For this review, take the finished solid that the model builds, in its own axes (mm). Face numbers are marked on the shaded views. A direction names the side the tool comes from. Round coordinates to 2 decimals unless told otherwise and drop trailing zeros. Loops run counter-clockwise (first coordinate to the right, second up) from the corner with the lowest first, then second, coordinate; pieces in that order, holes last.
1. Consider section B-B on x = 5. State the section outline as (y, z) points, then the cut area to 3 significant figures.
2. Consider section A-A on y = 4. State the section outline as (x, z) points.
3. Clearance check with flat-ended pins moving along their axes: pin 1 Ø1.9 at (x, z) = (11, 2.5) entering from +Y; pin 2 Ø1.9 at (y, z) = (-38.5, 2.5) entering from -X; pin 3 Ø2 at (x, y) = (83, -19.5) entering from +Z; pin 4 Ø1 at (x, z) = (44.5, 3) entering from +Y. State where each tip first meets the part, or that it passes through.
4. To check wall thickness, follow line 1 along Y through (x, z) = (103.75, 0.25); line 2 along Z through (x, y) = (98, 2); line 3 along Y through (x, z) = (84, 2.75). State the ranges of each line that lie inside material, in increasing order.
5. Tool access review of the marked faces 1 and 2: name each direction out of +Z, -Z, +X, -X, +Y, -Y from which nothing blocks a thin tool from reaching the whole face with its end or side.
6. Consider section C-C on y = -37. State how many separate pieces and enclosed holes the cut face has, then the cut area to 3 significant figures.
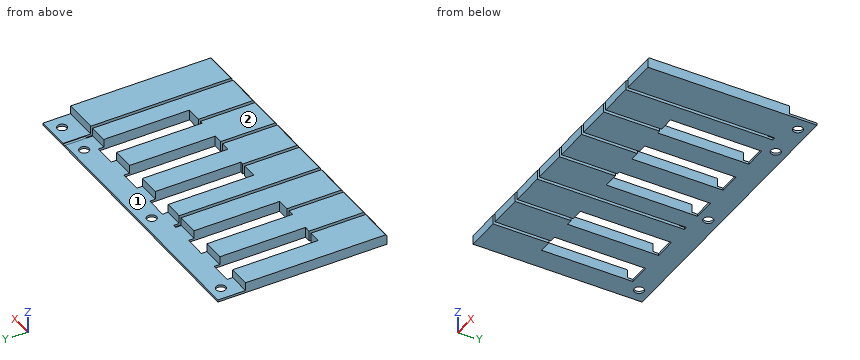
from build123d import *

# Parameters (mm, degrees)
PAD_DEPTH       = 0.81
SKETCH001_W     = 12.5
SKETCH001_H     = 51.2
PAD001_DEPTH    = 3
SKETCH002_R     = 1.75
POCKET_DEPTH    = 5
SKETCH003_W     = 1.25
SKETCH003_H     = 8
POCKET001_DEPTH = 0.2
CHAMFER_SIZE    = 0.5


with BuildPart() as part:
    # Sketch → Pad (new body)
    with BuildSketch(Plane.XY):
        Polygon((0, 0), (0, -53.2), (12.5, -53.2), (12.5, -33), (8, -33), (8, 0), (16, 0), (16, -33), (13.75, -33), (13.75, -53.2), (26.25, -53.2), (26.25, -33), (24, -33), (24, 0), (32, 0), (32, -33), (27.5, -33), (27.5, -53.2), (40, -53.2), (40, 0), (41.25, 0), (41.25, -53.2), (53.75, -53.2), (53.75, -33), (48.125, -33), (48.125, 0), (56.125, 0), (56.125, -33), (55, -33), (55, -53.2), (67.5, -53.2), (67.5, -33), (64.125, -33), (64.125, 0), (72.125, 0), (72.125, -33), (68.75, -33), (68.75, -53.2), (81.25, -53.2), (81.25, -33), (80.125, -33), (80.125, 0), (88.125, 0), (88.125, -33), (82.5, -33), (82.5, -53.2), (95, -53.2), (95, 0), (96.25, 0), (96.25, -53.2), (108.75, -53.2), (108.75, 0), (108.75, 8), (0, 8), align=None)
    extrude(amount=PAD_DEPTH)

    # Sketch001 (on Face56 of Pad) → Pad001 (join)
    with BuildSketch(Plane.XY.offset(0.81)):
        Polygon((0, -2), (0, -53.2), (12.5, -53.2), (12.5, -33), (8, -33), (8, -2), align=None)
        Polygon((16, -2), (16, -33), (13.75, -33), (13.75, -53.2), (26.25, -53.2), (26.25, -33), (24, -33), (24, -2), align=None)
        Polygon((32, -2), (32, -33), (27.5, -33), (27.5, -53.2), (40, -53.2), (40, -2), align=None)
        Polygon((41.25, -2), (41.25, -53.2), (53.75, -53.2), (53.75, -33), (48.125, -33), (48.125, -2), align=None)
        Polygon((56.125, -2), (56.125, -33), (55, -33), (55, -53.2), (67.5, -53.2), (67.5, -33), (64.125, -33), (64.125, -2), align=None)
        Polygon((72.125, -2), (72.125, -33), (68.75, -33), (68.75, -53.2), (81.25, -53.2), (81.25, -33), (80.125, -33), (80.125, -2), align=None)
        Polygon((88.125, -2), (88.125, -33), (82.5, -33), (82.5, -53.2), (95, -53.2), (95, -2), align=None)
        with Locations((102.5, -27.6)):
            Rectangle(SKETCH001_W, SKETCH001_H)
    extrude(amount=PAD001_DEPTH)

    # Sketch002 (on Face5 of Pad001) → Pocket (cut)
    with BuildSketch(Plane.XY.offset(0.81)):
        with Locations((5, 4)):
            Circle(SKETCH002_R)
        with Locations((48, 4)):
            Circle(SKETCH002_R)
        with Locations((90, 4)):
            Circle(SKETCH002_R)
        with Locations((103.75, 4)):
            Circle(SKETCH002_R)
    extrude(amount=-POCKET_DEPTH, mode=Mode.SUBTRACT)

    # Sketch003 (on Face5 of Pocket) → Pocket001 (cut)
    with BuildSketch(Plane.XY.offset(0.81)):
        with Locations((95.625, 4)):
            Rectangle(SKETCH003_W, SKETCH003_H)
    extrude(amount=-POCKET001_DEPTH, mode=Mode.SUBTRACT)

    # Chamfer
    chamfer_edges = [part.edges().sort_by_distance(p)[0] for p in [
        (6.25, -53.2, 3.81),
        (20, -53.2, 3.81),
        (33.75, -53.2, 3.81),
        (47.5, -53.2, 3.81),
        (61.25, -53.2, 3.81),
        (75, -53.2, 3.81),
        (88.75, -53.2, 3.81),
        (102.5, -53.2, 3.81),
    ]]
    chamfer(chamfer_edges, length=CHAMFER_SIZE)


solid = part.part
Resolved:
1. outline: (-53.2, 0) - (2.25, 0) - (2.25, 0.81) - (-2, 0.81) - (-2, 3.81) - (-52.7, 3.81) - (-53.2, 3.31) - close; (5.75, 0) - (8, 0) - (8, 0.81) - (5.75, 0.81) - close
1. area: 200 mm2
2. outline: (0, 0) - (3.25, 0) - (3.25, 0.81) - (0, 0.81) - close; (6.75, 0) - (46.25, 0) - (46.25, 0.81) - (6.75, 0.81) - close; (49.75, 0) - (88.25, 0) - (88.25, 0.81) - (49.75, 0.81) - close; (91.75, 0) - (102, 0) - (102, 0.81) - (96.25, 0.81) - (96.25, 0.61) - (95, 0.61) - (95, 0.81) - (91.75, 0.81) - close; (105.5, 0) - (108.75, 0) - (108.75, 0.81) - (105.5, 0.81) - close
3. pin 1: stops at y = -33
3. pin 2: stops at x = 0
3. pin 3: passes through
3. pin 4: stops at y = -2
4. line 1: y = -53.2 to 2.25, 5.75 to 8
4. line 2: z = 0 to 0.81
4. line 3: y = -53.2 to -33
5. face 1: +Z, +X, -X, +Y
5. face 2: +Z, +X, -X, +Y, -Y
6. separate pieces: 8
6. enclosed holes: 0
6. area: 381 mm2
